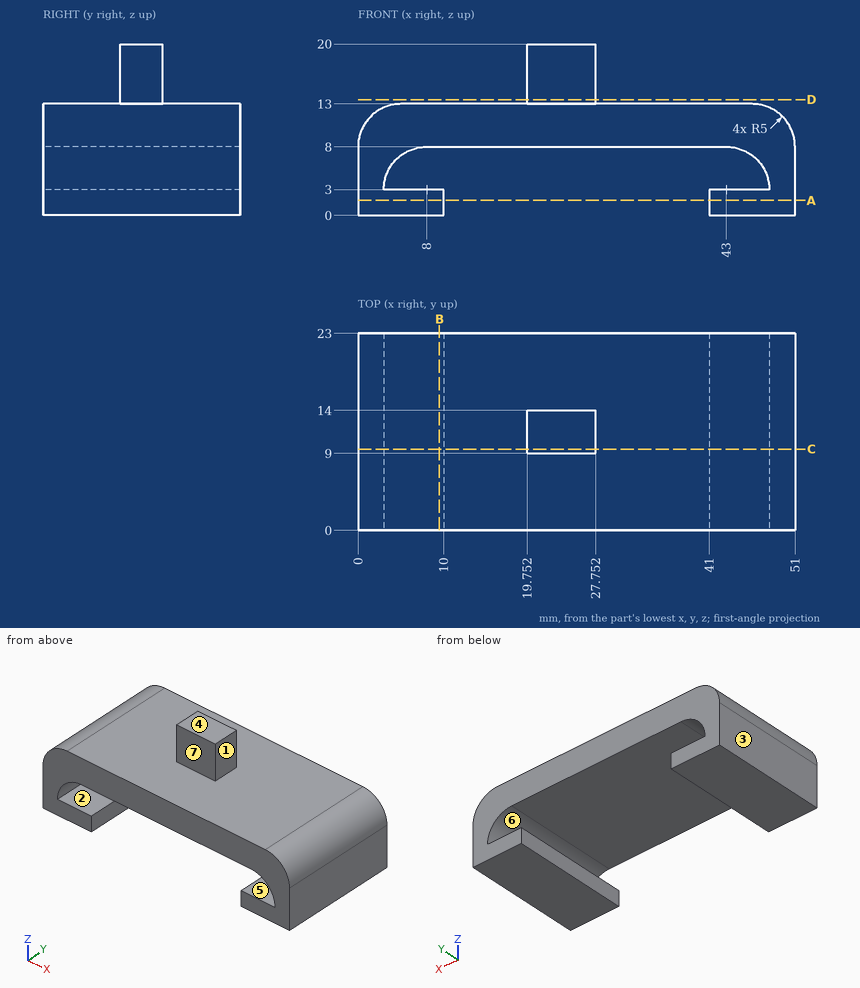
Study the drawing (mm; zero at the part's minimum x, y, z) and answer. A direction names the side the tool comes from. Coordinates: 2 decimals unless noted, no trailing zeros. Order: outer loops, then holes, each group sorted by start corner. A loop starts at its lowest first (then second) coordinate and runs counter-clockwise, first axis right, second up. Notation, with made-up numbers: M -15.5,54 L 42.5,54 A16 cw 42.5,84 Z; hole C 0,8.25 d4. An arc over 180 degrees is marked long. Use CSV: the item, a comma, the result in double quotes.
Q1. Section D-D (z = 13.5) is taken. Determine the outline of the cut face in (x, y), then the cut area to 3 significant figures.
Here are the results:
outline,"M 19.75,9 L 27.75,9 L 27.75,14 L 19.75,14 Z"
area,"40.0 mm2"
Q2. Section A-A (z = 1.75) is taken. Determine the outline of the cut face in (x, y).
Here are the results:
outline,"M 0,0 L 10,0 L 10,23 L 0,23 Z; M 41,0 L 51,0 L 51,23 L 41,23 Z"
Q3. A tool of negligible diameter and unlimited length cuts with its end or side. For the marked faces 1, 2 and 3, from which of +Z, -Z, +X, -X, +Y, -Y can it reach the whole face along a straight path? Write none if from no direction.
Here are the results:
face 1,"+Z, +X, +Y, -Y"
face 2,"+Y, -Y"
face 3,"+Z, -Z, -X, +Y, -Y"
Q4. Section C-C (y = 9.5) is taken. Determine the outline of the cut face in (x, z), then the cut area to 3 significant figures.
Here are the results:
outline,"M 0,0 L 10,0 L 10,3 L 3,3 A5 cw 8,8 L 43,8 A5 cw 48,3 L 41,3 L 41,0 L 51,0 L 51,8 A5 ccw 46,13 L 27.75,13 L 27.75,20 L 19.75,20 L 19.75,13 L 5,13 A5 ccw 0,8 Z"
area,"401 mm2"
Q5. Straight lines are drawn through the part: L1, parallel to X at y = 2, z = 7; L2, parallel to X at y = 3.75, z = 2.25; L3, parallel to Z at x = 33, y = 7. For each, find the intervals that lie inside material, in ascending order.
Here are the results:
L1,"0 to 5, 46 to 51"
L2,"0 to 10, 41 to 51"
L3,"8 to 13"
Q6. Determine the mould class of the marked faces 4, 5, 6 and 7 for opening direction Z: pulls with the +Z half, pulls with the -Z half, needs draft (parallel to the pull), parting line crosses it, or undercut.
Here are the results:
face 4,"pulls with the +Z half"
face 5,"undercut"
face 6,"undercut"
face 7,"needs draft"
Q7. Section B-B (x = 9.5) is taken. Determine the outline of the cut face in (y, z), then the cut area to 3 significant figures.
Here are the results:
outline,"M 0,0 L 23,0 L 23,3 L 0,3 Z; M 0,8 L 23,8 L 23,13 L 0,13 Z"
area,"184 mm2"
Q8. Given pin 1 Ø7.5 at (x, z) = (24, 18) entering from -Y; pin 2 Ø1.5 at (y, z) = (12, 18) entering from -X; pin 3 Ø2 at (y, z) = (9, 13) entering from -X, each flat-ended and moving along its own axis, determine where each tip first touches the part or whether it passes through.
Here are the results:
pin 1,"y = 9"
pin 2,"x = 19.75"
pin 3,"x = 2"
